from build123d import *

# Parameters (mm, degrees)
F0_W     = 627.888
F0_H     = 38.1
F1_DEPTH = 19.05
F3_DEPTH = 38.101
F4_R     = 5.08


with BuildPart() as f1:
    # F0 (on Front) → F1 (new body, symmetric)
    with BuildSketch(Plane.XZ):
        Rectangle(F0_W, F0_H)
    extrude(amount=F1_DEPTH, both=True)

    # F2 (on face) → F3 (cut, through all)
    with BuildSketch(Plane.XZ.offset(19.05)):
        Polygon((313.944, 19.05), (271.231802, 19.05), (263.133398, -19.05), (313.944, -19.05), align=None)
    extrude(amount=-F3_DEPTH, mode=Mode.SUBTRACT)

    # F4
    f4_edges = [f1.edges().sort_by_distance(p)[0] for p in [
        (-21.356099, -19.05, 19.05),
        (-25.405301, -19.05, -19.05),
        (-21.356099, 19.05, 19.05),
        (-25.405301, 19.05, -19.05),
    ]]
    fillet(f4_edges, radius=F4_R)


solid = f1.part
Geometry: final body of the model. Coordinates: model frame, mm. Round coordinates to 2 decimals unless told otherwise and drop trailing zeros. Loops run counter-clockwise (first coordinate to the right, second up) from the corner with the lowest first, then second, coordinate; pieces in that order, holes last.
Q1. Pin query (flat end, axial travel): P1, Ø3, axis at y = -9, z = -10, coming from the +X side; P2, Ø1, axis at y = 2, z = 10.5, coming from the +X side; P3, Ø10, axis at y = 12, z = -7, coming from the +X side. Return the tip coordinate at first contact, or that it passes through.
Q2. Section A-A on x = -161.5. Return loops of the section in (y, z).
Q3. Material intervals for L1, parallel to Y at x = -162.5, z = 15; L2, parallel to X at y = -14.5, z = 15; L3, parallel to X at y = -7, z = -11.5, sorted ascending.
Evaluation:
1. P1: stops at x = 265.38
1. P2: stops at x = 269.52
1. P3: stops at x = 266.76
2. outline: (-19.05, -13.97) arc R5.08 ccw to (-13.97, -19.05) - (13.97, -19.05) arc R5.08 ccw to (19.05, -13.97) - (19.05, 13.97) arc R5.08 ccw to (13.97, 19.05) - (-13.97, 19.05) arc R5.08 ccw to (-19.05, 13.97) - close
3. L1: y = -18.94 to 18.94
3. L2: x = -313.94 to 270.37
3. L3: x = -313.94 to 264.74
